Autodesk Inventor part; units mm, degrees
ref_plane "Arbeitsebene1" through (0, 1.2, 0) normal (0, 1, 0) x (-1, 0, 0)
ref_plane "YZ Plane" through (0, 0, 0) normal (1, 0, 0) x (0, 1, 0)
ref_plane "XY Plane" through (0, 0, 0) normal (0, 0, 1) x (1, 0, 0)
sketch "Skizze1" plane through (0, 0, 0) normal (0, 0, 1) x (1, 0, 0)
  line L0 (42, 1) -> (0, 1)
  line L1 (0, 2.25) -> (0, 1)
  arc A0 (0.25, 2.5) -> (0, 2.25) centre (0.25, 2.25) ccw
  line L2 (0.25, 2.5) -> (12, 2.5)
  line L3 (12, 1.75) -> (12, 2.5)
  line L4 (34, 1) -> (34, 0.995)
  line L5 (-8.4621, 0) -> (50.4104, 0)
  line L6 (0, 0.6836) -> (0, 2.8631)
  line L7 (11.9997, 1.75) -> (39.9817, 1.75)
  line L8 (42, 1) -> (42, 1.284)
  line L9 (42, 1.284) -> (39.9817, 1.75)
  dimension "d0" = 2
  dimension "d1" = 5
  dimension "d8" = 42
  dimension "d9" = 0.25
  dimension "d10" = 3.5
  dimension "d24" = 103
revolve "Umdrehung1" add sketch "Skizze1" angle 360 about axis through (-10, 0, 0) along (1, 0, 0)
ref_plane "Arbeitsebene1" through (0, 1.2, 0) normal (0, 1, 0) x (-1, 0, 0)
sketch "Skizze2" plane through (0, 1.2, 0) normal (0, 1, 0) x (-1, 0, 0)
  line L0 (8.4, 0) -> (-50.4, 0)
  arc A0 (-10.3, 1.5) -> (-10.3, -1.5) centre (-10.3, 0) ccw
  line L1 (0, 1) -> (0, -1)
  line L2 (-10.3, -1.5) -> (0, -1.5)
  line L3 (-42, -1) -> (0, -1)
  line L4 (-10.3, 1.5) -> (0, 1.5)
  line L5 (0, 2.25) -> (0, -2.25)
  line L6 (0, 1.5) -> (0, -1.5)
  point P0 (0, 0)
  dimension "d13" = 3
  dimension "d14" = 10.3
extrude "Extrusion1" cut sketch "Skizze2" along normal through all
sketch "Skizze3" plane through (0, 0, 0) normal (0, 0, 1) x (1, 0, 0)
  line L0 (-8.4, 0) -> (50.4, 0)
  line L1 (42, 0.1) -> (34, 0.1)
  line L2 (34, 0.1) -> (34, -0.1)
  line L3 (34, -0.1) -> (42, -0.1)
  line L4 (42, -0.1) -> (42, 0.1)
  line L5 (42, -1) -> (42, 1)
  point P0 (0, 0)
  dimension "d17" = 8
  dimension "d18" = 0.2
extrude "Extrusion2" cut sketch "Skizze3" along normal through all both and the other way through all
pattern_circular "Runde Anordnung1" count 4 over 360 about axis through (25.9908, 0, 0) along (1, 0, 0) of "Extrusion2"
thread "Gewinde1"
fillet "Rundung1" radius 0.2 2 edges at (12, -1.75, 0) (12, -2.5, 0)
fillet "Rundung2" radius 0.1 3 edges at (11.8, 1.2, 0) (5.15, 1.2, 1.5) (5.15, 1.2, -1.5)
properties part number "YTP-AP-E14-R1.0"
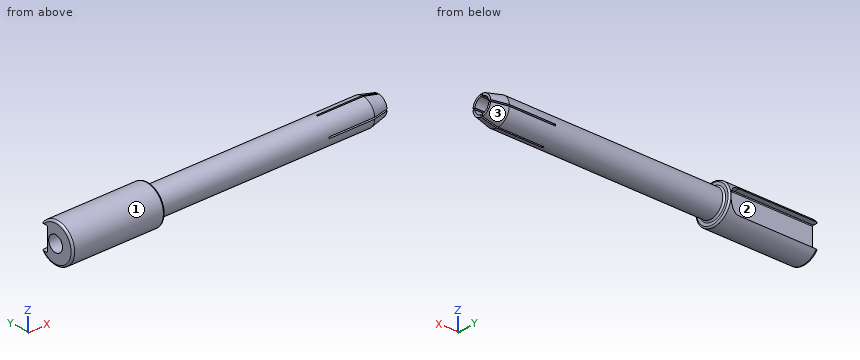
Build history of the part. All positions in model axes, mm. Face numbers are marked on the shaded views. Give positions to 0.01 mm unless a question says otherwise; leave off trailing zeros. Loops run counter-clockwise (first coordinate to the right, second up) from the corner with the lowest first, then second, coordinate; pieces in that order, holes last. Notation, with made-up numbers: (73.5, 79) -> (113.5, 79) arc R21 cw to (113.5, 103) -> close; hole circle Ø1 at (47.5, 38.5). An arc over 180 degrees is marked (long way). One line per question, with ' | ' between items. Start each with the question number.
1) Cut at A-A (x = 6). Give the cut face in (y, z).
2) Pin check, flat tips, straight feed: pin 1 (2 mm diameter, centred on x = 37, y = 1, fed in from +Z); pin 2 (3 mm diameter, centred on x = 33, y = 0.5, fed in from +Z); pin 3 (1.4 mm diameter, centred on x = 5.5, z = 0, fed in from +Y). Stop position of each tip, or through.
3) Probe L1, parallel to Z at x = 16, y = 0; L2, parallel to Y at x = 9, z = 0; L3, parallel to Y at x = 9, z = 0.35. List the from-to ranges inside material, lowest first.
4) Cut at B-B (x = 17). Give the cut face in (y, z).
5) Two-plate mould, pull along Z, no slides. Class the marked faces 1, 2 and 3: released by +Z, released by -Z, zero draft, split by the parting line, or undercut.
Return value:
1) outline: (1.2, -1.4) -> (1.2, 1.4) arc R0.1 cw to (1.3, 1.5) -> (2, 1.5) arc R2.5 ccw (long way) to (2, -1.5) -> (1.3, -1.5) arc R0.1 cw to start; hole circle Ø2 at (0, 0)
2) pin 1: z = 1.75 | pin 2: z = 1.75 | pin 3: y = 1.2
3) L1: -1.75 to -1, 1 to 1.75 | L2: -2.5 to -1, 1 to 1.2 | L3: -2.48 to -0.94, 0.94 to 1.2
4) outline: circle Ø3.5 at (0, 0); hole circle Ø2 at (0, 0)
5) face 1: split by the parting line | face 2: undercut | face 3: released by -Z
